Input: part model. Units: mm. Frame: model coordinates. A direction names the side the tool comes from. Coordinates: 2 decimals unless noted, no trailing zeros. Write each loop counter-clockwise with the first axis right and the second up, starting at its lowest first coordinate (ties: lowest second). Pieces come first, ordered by that corner, then holes. Notation, with made-up numbers: (8.25, 21) - (22.25, 21) arc R4 cw to (22.25, 25) - close; hole circle Ø7 at (46, 42). An arc over 180 degrees is marked (long way). One line per question, with ' | ' between items. Start each with the question number.
1) Section query D-D on y = 13.5. Return loops of the section in (x, z).
2) Section query A-A on z = 12. Return loops of the section in (x, y), and give its area (3 significant figures).
3) Reachability of faces 4 (the flat face through (-17.059, 31, 17)), 5 (the flat face through (-24, -9, 0)), 6 (the flat face through (-24, -9, 20)), 7 (the flat face through (44, 6, 8)), 8 (the flat face through (43.4, -6, 7.6)) from +Z, -Z, +X, -X, +Y, -Y: full face, straight path, thin tool, end or side. Return the list, or none.
4) Section query C-C on x = 30.5. Return loops of the section in (y, z), and give its area (3 significant figures).
5) Section query B-B on y = 22. Return loops of the section in (x, z), and give its area (3 significant figures).
6) First-contact query: P1, Ø10, axis at x = 27.5, z = 14, coming from the -Y side; P2, Ø7, axis at x = -9.06, y = 33.81, coming from the -Z side; P3, Ø10, axis at x = 23.5, y = -16, coming from the -Z side; P4, Ø1.5, axis at x = -7, z = 3.5, coming from the -Y side. Flat tips, straight axial feed; report the tip coordinate or a pass-through.
7) Draft query along Y for faces 1 (the cylindrical face through (2.66, -30.46, 17.54)), 2 (the cylindrical face through (47.15, -3.46, 16.99)), 3 (the flat face through (35, 1, 10)). Return one class per face: released by +Y, released by -Y, zero draft, split by the parting line, or undercut.
8) Line query: line 1 (X direction, y = -4.5, z = 10); line 2 (Z direction, x = 14, y = 24.5); line 3 (X direction, y = -4.15, z = 10). Output: solid intervals per line, ascending.
```python
from build123d import *

# Parameters (mm, degrees)
SKETCH1_R              = 4
BOSS_EXTRUDE1_DEPTH    = 20
FILLET1_R              = 10
CUT_EXTRUDE1_START     = -41.80740392
CUT_EXTRUDE1_OUTLINE_R = 4
CUT_EXTRUDE1_DEPTH     = 83.61480784
FILLET2_R              = 5


# Read off the part's stored shape, not the designer's step: Cut-Extrude1
with BuildPart() as part:
    # Sketch1 → Boss-Extrude1 (new body)
    with BuildSketch(Plane(origin=(0, 0, 0), x_dir=(0, 1, 0), z_dir=(0, 0, 1))):
        with BuildLine():
            ThreePointArc((24.677963744, 17.058666579), (0, 30), (-24.677963744, 17.058666579))
            Line((-24.677963744, 17.058666579), (-33.80740392, 17.058666579))
            ThreePointArc((-33.80740392, 17.058666579), (-41.534810495, 11.129219073), (-37.80740416, 2.130463487))
            Line((-37.80740416, 2.130463487), (-29.901076805, -2.43425674))
            ThreePointArc((-29.901076805, -2.43425674), (-22.448320849, -19.901580115), (-6, -29.393876913))
            Line((-6, -29.393876913), (-6, -50))
            Line((-6, -50), (-1, -50))
            Line((-1, -50), (-1, -24.979991994))
            ThreePointArc((-1, -24.979991994), (0, 25), (1, -24.979991994))
            Line((1, -24.979991994), (1, -50))
            Line((1, -50), (6, -50))
            Line((6, -50), (6, -29.393876913))
            ThreePointArc((6, -29.393876913), (22.448320849, -19.901580115), (29.901076805, -2.43425674))
            Line((29.901076805, -2.43425674), (37.807403702, 2.130463222))
            ThreePointArc((37.807403702, 2.130463222), (41.534810563, 11.129218818), (33.80740392, 17.058666579))
            Line((33.80740392, 17.058666579), (24.677963744, 17.058666579))
        make_face()
        with Locations(Location((-33.80740392, 9.058666579, 0), (0, 0, 270))):
            Circle(SKETCH1_R, mode=Mode.SUBTRACT)
        with Locations(Location((33.80740392, 9.058666579, 0), (0, 0, 270))):
            Circle(SKETCH1_R, mode=Mode.SUBTRACT)
    extrude(amount=BOSS_EXTRUDE1_DEPTH)

    # Fillet1
    fillet1_edges = [part.edges().sort_by_distance(p)[0] for p in [
        (50, 3.5, 0),
        (50, 3.5, 20),
        (50, -3.5, 0),
        (50, -3.5, 20),
    ]]
    fillet(fillet1_edges, radius=FILLET1_R - 0.0001)  # a hair under: the kernel refuses the full size

    # Cut-Extrude1 outline → Cut-Extrude1 (cut)
    with BuildSketch(Plane(origin=(0, 0, 0), x_dir=(-1, 0, 0), z_dir=(0, 1, 0)).offset(CUT_EXTRUDE1_START)):
        with BuildLine():
            ThreePointArc((17.5, 5), (22.5, 10), (17.5, 15))
            Line((17.5, 15), (-17.5, 15))
            ThreePointArc((-17.5, 15), (-22.5, 10), (-17.5, 5))
            Line((-17.5, 5), (17.5, 5))
        make_face()
        with Locations((-40, 10)):
            Circle(CUT_EXTRUDE1_OUTLINE_R)
    extrude(amount=CUT_EXTRUDE1_DEPTH, mode=Mode.SUBTRACT)

    # Fillet2
    fillet2_edges = [part.edges().sort_by_distance(p)[0] for p in [
        (29.393876913, -6, 10),
        (2.43425674, -29.901076805, 17.5),
        (2.43425674, -29.901076805, 2.5),
        (-17.058666579, -24.677963744, 17.5),
        (-17.058666579, -24.677963744, 2.5),
        (-17.058666579, 24.677963744, 17.5),
        (-17.058666579, 24.677963744, 2.5),
        (2.43425674, 29.901076805, 2.5),
        (2.43425674, 29.901076805, 17.5),
        (29.393876913, 6, 10),
    ]]
    fillet(fillet2_edges, radius=FILLET2_R)


solid = part.part
```
Answer key:
1) outline: (-26.79, 0) - (-21.04, 0) - (-21.04, 6.47) arc R5 cw to (-21.04, 13.53) - (-21.04, 20) - (-26.79, 20) - close; (21.04, 0) - (26.79, 0) - (26.79, 20) - (21.04, 20) - (21.04, 13.53) arc R5 cw to (21.04, 6.47) - close
2) outline: (-22.08, -20.31) - (-22.08, -11.72) arc R25 cw to (-22.08, 11.72) - (-22.08, 20.31) arc R30 ccw to start; (22.08, -20.31) arc R30 ccw to (28.48, -9.43) arc R5 cw to (33.23, -6) - (36.54, -6) - (36.54, -1) - (24.98, -1) arc R25 cw to (22.08, -11.72) - close; (22.08, 11.72) arc R25 cw to (24.98, 1) - (36.54, 1) - (36.54, 6) - (33.23, 6) arc R5 cw to (28.48, 9.43) arc R30 ccw to (22.08, 20.31) - close; (43.46, -6) - (49.8, -6) - (49.8, -1) - (43.46, -1) - close; (43.46, 1) - (49.8, 1) - (49.8, 6) - (43.46, 6) - close | area: 476 mm²
3) face 4: +Z, -Z, -X, +Y | face 5: -Z, +X, -X, +Y, -Y | face 6: +Z, +X, -X, +Y, -Y | face 7: +Z, -Z, +X, +Y | face 8: +Z, -Z, +X, -Y
4) outline: (-6.81, 0) - (-1, 0) - (-1, 20) - (-6.81, 20) - close; (1, 0) - (6.81, 0) - (6.81, 20) - (1, 20) - close | area: 232 mm²
5) outline: (-20.4, 0) - (-11.87, 0) - (-11.87, 5) - (-17.5, 5) arc R5 cw to (-20.4, 5.92) - close; (-20.4, 14.08) arc R5 cw to (-17.5, 15) - (-11.87, 15) - (-11.87, 20) - (-20.4, 20) - close; (11.87, 0) - (20.4, 0) - (20.4, 5.92) arc R5 cw to (17.5, 5) - (11.87, 5) - close; (11.87, 15) - (17.5, 15) arc R5 cw to (20.4, 14.08) - (20.4, 20) - (11.87, 20) - close | area: 174 mm²
6) P1: y = -19.84 | P2: through | P3: z = 0 | P4: y = -41.7
7) face 1: released by -Y | face 2: zero draft | face 3: undercut
8) line 1: -29.66 to -24.59, 24.59 to 36, 44 to 50 | line 2: 0 to 5, 15 to 20 | line 3: -29.71 to -24.65, 24.65 to 36, 44 to 50
